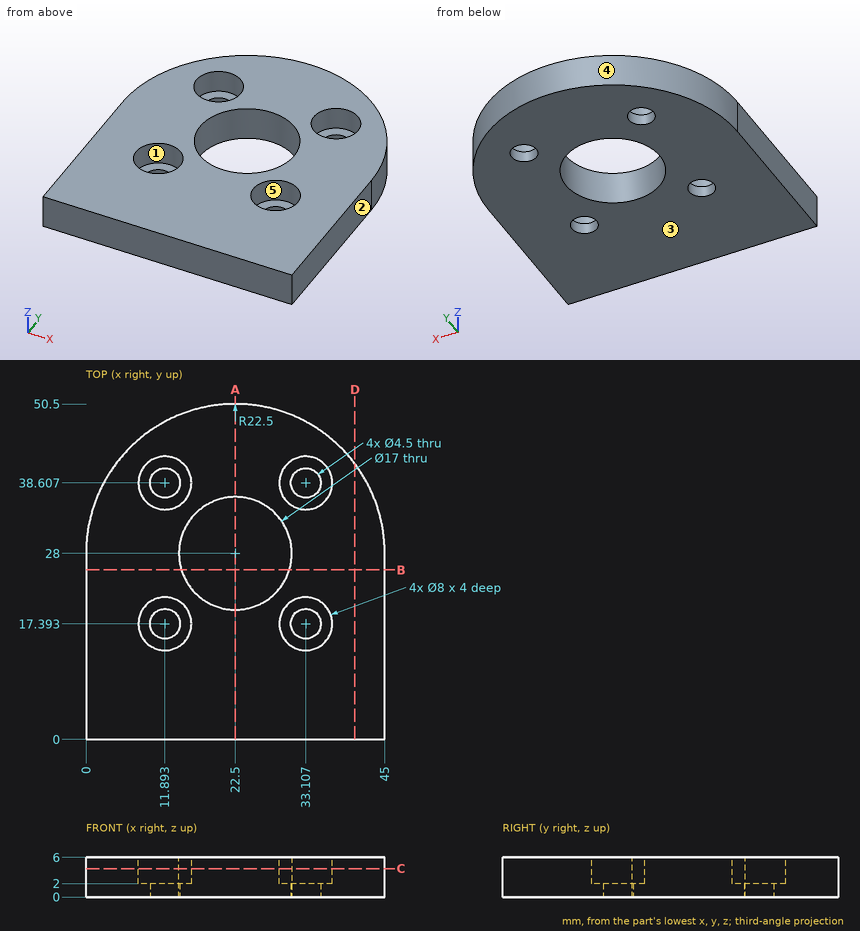
Study the drawing (mm; zero at the part's minimum x, y, z) and answer. A direction names the side the tool comes from. Coordinates: 2 decimals unless noted, no trailing zeros. Loops run counter-clockwise (first coordinate to the right, second up) from the corner with the lowest first, then second, coordinate; pieces in that order, holes last. Notation, with made-up numbers: (80, 61) -> (121, 61) arc R24 ccw to (121, 92) -> close; hole circle Ø8 at (14.5, -23). An arc over 180 degrees is marked (long way). Write item = value, one per line. Start each with the question number.
1) For the marked faces 1 and 2, determine the directions among +Z, -Z, +X, -X, +Y, -Y from which every point of the face is accessible in a straight line to the end or side of a thin tool.
2) Given P1, Ø2.5, axis at x = 12.5, y = 16, coming from the +Z side; P2, Ø1, axis at x = 16.5, z = 2, coming from the +Y side; P3, Ø1.5, axis at y = 32.5, z = 1, coming from the -X side (1 decimal), each flat-ended and moving along its own axis, determine where each tip first touches the part or whether it passes through.
3) The part is cut by section D-D, the plane x = 40.5. Determine the outline of the cut face in (y, z), plus the area to 3 significant figures.
4) The part is cut by section C-C, the plane z = 4.3. Determine the outline of the cut face in (x, y), plus the area to 3 significant figures.
5) The mould has two halves that part along Y. Classify the marked faces 3, 4 and 5: pulls with the +Y half, pulls with the -Y half, needs draft (parallel to the pull), parting line crosses it, or undercut.
6) The part is cut by section A-A, the plane x = 22.5. Determine the outline of the cut face in (y, z), plus the area to 3 significant figures.
7) The part is cut by section B-B, the plane y = 25.5. Determine the outline of the cut face in (x, z).
8) Find the intervals of material crossed by L1, parallel to X at y = 40, z = 1.15 (1 decimal); L2, parallel to X at y = 38, z = 5.1 (1 decimal); L3, parallel to Y at x = 15, z = 5.2 (1 decimal), in increasing order. Write a range as from..to.
Result:
q1.face_1 = +Z
q1.face_2 = +Z, -Z, +X, +Y, -Y
q2.P1 = 2
q2.P2 = 49.82
q2.P3 = 0.3
q3.outline = (0, 0) -> (41.5, 0) -> (41.5, 6) -> (0, 6) -> close
q3.area = 249 mm²
q4.outline = (0, 0) -> (45, 0) -> (45, 28) arc R22.5 ccw to (0, 28) -> close; hole circle Ø8 at (11.89, 17.39); hole circle Ø8 at (11.89, 38.61); hole circle Ø17 at (22.5, 28); hole circle Ø8 at (33.11, 17.39); hole circle Ø8 at (33.11, 38.61)
q4.area = 1,630 mm²
q5.face_3 = needs draft
q5.face_4 = pulls with the +Y half
q5.face_5 = undercut
q6.outline = (0, 0) -> (19.5, 0) -> (19.5, 6) -> (0, 6) -> close; (36.5, 0) -> (50.5, 0) -> (50.5, 6) -> (36.5, 6) -> close
q6.area = 201 mm²
q7.outline = (0, 0) -> (14.38, 0) -> (14.38, 6) -> (0, 6) -> close; (30.62, 0) -> (45, 0) -> (45, 6) -> (30.62, 6) -> close
q8.L1 = 3.5..10.1, 13.7..31.3, 34.9..41.5
q8.L2 = 2.3..7.9, 15.8..29.2, 37.1..42.7
q8.L3 = 0..14.9, 19.9..24, 32..36.1, 41.1..49.2
